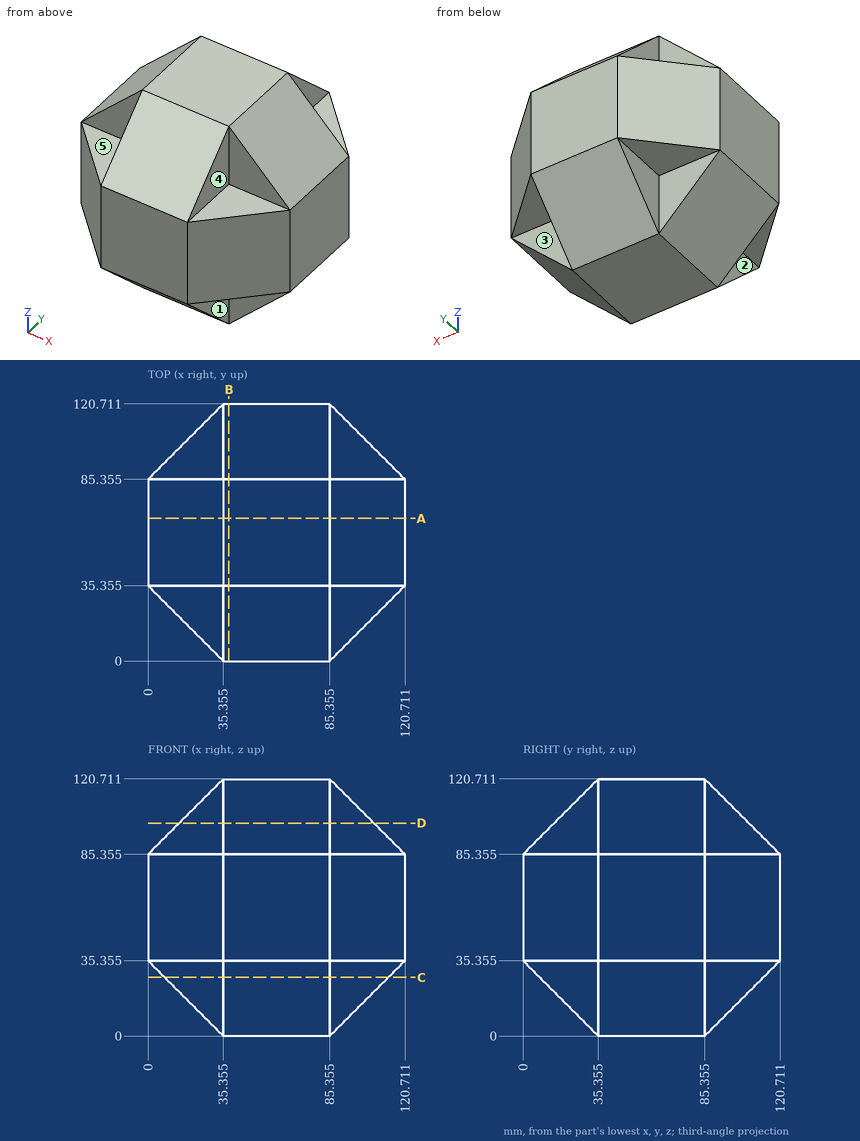
Print and shaded views of the part. All mm, measured from the part's lowest x, y and z. A direction names the side the tool comes from. Give positions to 0.01 mm unless a question says otherwise; leave off trailing zeros. Write each loop counter-clockwise with the first axis right and the second up, starting at its lowest first coordinate (ties: lowest second). Pieces come first, ordered by that corner, then holes. Notation, with made-up numbers: (21.5, 20.5) - (70.5, 20.5) arc R3 cw to (70.5, 24.5) - close; hole circle Ø3 at (-19, -3). An arc over 180 degrees is marked (long way). One line per question, with ' | ' between items. Start each with the question number.
(1) 3-axis set-ups, long thin cutter, end or side, ignore diameter. For the marked faces 1, 2, 3, 4 and 5: which of +Z, -Z, +X, -X, +Y, -Y reach the whole face in a straight line?
(2) Slice it at D-D on z = 100. Write the cut outline in (x, y) (1 decimal).
(3) Slice it at C-C on z = 27.5. Write the cut outline in (x, y) (1 decimal), plus the area to 3 significant figures.
(4) Slice it at A-A on y = 67. Write the cut outline in (x, z) (1 decimal), plus the area to 3 significant figures.
(5) Pin check, flat tips, straight feed: P1, Ø17.5, axis at x = 12.5, z = 95.5, coming from the +Y side (1 decimal); P2, Ø6, axis at x = 100, z = 52, coming from the -Y side (1 decimal); P3, Ø2, axis at x = 37.5, y = 14.5, coming from the -Z side (1 decimal). Stop position of each tip, or through.
(6) Wall check: line 1 along X through (y, z) = (24, 92.5) (1 decimal). Give the ranges that are in metal, low to high. Write a range as from..to.
Results below:
1) face 1: -Z, +X, -Y | face 2: -Z, -X, -Y | face 3: -Z, +X, +Y | face 4: +Z, +X, -Y | face 5: +Z, -X, -Y
2) outline: (14.6, 35.4) - (35.4, 35.4) - (35.4, 14.6) - (85.4, 14.6) - (85.4, 35.4) - (106.1, 35.4) - (106.1, 85.4) - (85.4, 85.4) - (85.4, 106.1) - (35.4, 106.1) - (35.4, 85.4) - (14.6, 85.4) - close
3) outline: (7.9, 35.4) - (35.4, 35.4) - (35.4, 7.9) - (85.4, 7.9) - (85.4, 35.4) - (112.9, 35.4) - (112.9, 85.4) - (85.4, 85.4) - (85.4, 112.9) - (35.4, 112.9) - (35.4, 85.4) - (7.9, 85.4) - close | area: 8,000 mm^2
4) outline: (0, 35.4) - (35.4, 0) - (85.4, 0) - (120.7, 35.4) - (120.7, 85.4) - (85.4, 120.7) - (35.4, 120.7) - (0, 85.4) - close | area: 12,100 mm^2
5) P1: y = 85.4 | P2: y = 11.6 | P3: z = 19.9
6) line 1: 35.4..85.4
